Can you work these out from the model? Positions are in its coordinate system, mm. A direction names the side the tool comes from. Coordinates: 2 decimals unless noted, no trailing zeros. Order: outer loops, then holes, each group sorted by start corner. A loop starts at its lowest first (then second) coordinate and runs counter-clockwise, first axis right, second up. Notation, with made-up numbers: (70, -31) -> (121, -31) arc R25 ccw to (121, -11) -> close; hole circle Ø3 at (-24.75, 27.5). An arc over 180 degrees is marked (long way). Write item = value, one per line.
Autodesk Inventor part; units mm, degrees
ref_plane "YZ Plane" through (0, 0, 0) normal (1, 0, 0) x (0, 1, 0)
ref_plane "XZ Plane" through (0, 0, 0) normal (0, 1, 0) x (-1, 0, 0)
ref_plane "XY Plane" through (0, 0, 0) normal (0, 0, 1) x (1, 0, 0)
sketch "Sketch1" plane through (0, 0, 0) normal (0, 0, 1) x (1, 0, 0)
  line L0 (-81.5, 70) -> (81.5, 70)
  line L1 (81.5, 70) -> (81.5, -70)
  line L2 (81.5, -70) -> (-81.5, -70)
  line L3 (-81.5, -70) -> (-81.5, 70)
  line L4 (-81.5, 70) -> (81.5, -70) construction
  line L5 (81.5, 70) -> (-81.5, -70) construction
  line L6 (81.5, 62) -> (89.5, 62)
  line L7 (89.5, 62) -> (89.5, 44)
  line L8 (89.5, 44) -> (81.5, 44)
  line L9 (81.5, 44) -> (81.5, 62)
  line L10 (81.5, -58) -> (89.5, -58)
  line L11 (89.5, -58) -> (89.5, -40)
  line L12 (89.5, -40) -> (81.5, -40)
  line L13 (81.5, -40) -> (81.5, -58)
  line L14 (-81.5, 62) -> (-89.5, 62)
  line L15 (-89.5, 62) -> (-89.5, 44)
  line L16 (-89.5, 44) -> (-81.5, 44)
  line L17 (-81.5, 44) -> (-81.5, 62)
  line L18 (-81.5, -58) -> (-89.5, -58)
  line L19 (-89.5, -58) -> (-89.5, -40)
  line L20 (-89.5, -40) -> (-81.5, -40)
  line L21 (-81.5, -40) -> (-81.5, -58)
  point P0 (0, 0)
  dimension "d0" = 163
  dimension "d1" = 140
  dimension "d2" = 8
  dimension "d3" = 18
  dimension "d4" = 8
  dimension "d5" = 12
extrude "Extrusion1" add sketch "Sketch1" along normal blind 5
sketch "Sketch2" plane through (0, 0, 5) normal (0, 0, 1) x (1, 0, 0)
  line L0 (-80, -67) -> (80, -67)
  line L1 (80, -67) -> (80, 67)
  line L2 (80, 67) -> (-80, 67)
  line L3 (-80, 67) -> (-80, -67)
  line L4 (-80, -67) -> (80, 67) construction
  line L5 (80, -67) -> (-80, 67) construction
  line L6 (81.5, 70) -> (-81.5, 70)
  line L7 (81.5, -40) -> (81.5, 44)
  point P0 (0, 0)
  dimension "d48" = 160
  dimension "d49" = 134
extrude "Extrusion2" add sketch "Sketch2" along normal blind 11
sketch "Sketch3" plane through (0, 0, 0) normal (1, 0, 0) x (0, 1, 0)
  line L0 (49.75, 0) -> (-49.75, 0)
  line L1 (49.75, 0) -> (66.532, 20)
  line L2 (66.532, 20) -> (-66.532, 20)
  line L3 (-66.532, 20) -> (-49.75, 0)
  point P0 (0, 0)
  point P1 (0, 0)
  dimension "d12" = 99.5
  dimension "d13" = 20
  dimension "d14" = 130
  dimension "d15" = 130
extrude "Extrusion3" cut sketch "Sketch3" against normal mid plane 148
chamfer "Chamfer1" distance 2.82 angle 80 1 edges at (74, 0, 16) measured on face at (78, -21.0585, 16)
chamfer "Chamfer2" distance 2.82 angle 80 1 edges at (-74, 0, 16) measured on face at (-78, 21.0585, 16)
fillet "Fillet1" radius 4 4 edges at (-80, 67, 10.5) (-80, -67, 10.5) (80, 67, 10.5) (80, -67, 10.5)
fillet "Fillet3" radius 1 4 edges at (-75.41, -56.4657, 8.0035) (75.41, -56.4657, 8.0035) (75.41, 56.4657, 8.0035) (-75.41, 56.4657, 8.0035)
fillet "Fillet4" radius 3 8 edges at (89.5, 62, 2.5) (89.5, -40, 2.5) (89.5, -58, 2.5) (89.5, 44, 2.5) (-89.5, 62, 2.5) (-89.5, 44, 2.5) (-89.5, -40, 2.5) (-89.5, -58, 2.5)
fillet "Fillet5" radius 2 12 edges at (-81.5, 70, 2.5) (81.5, 70, 2.5) (-81.5, -70, 2.5) (81.5, -70, 2.5) (-81.5, -58, 2.5) (-81.5, 44, 2.5) (81.5, -40, 2.5) (81.5, -58, 2.5) (81.5, 62, 2.5) (-81.5, 62, 2.5) (-81.5, -40, 2.5) (81.5, 44, 2.5)
sketch "Sketch4" plane through (0, 0, 5) normal (0, 0, 1) x (1, 0, 0)
  line L0 (-84, -50.9) -> (84, -50.9)
  line L1 (84, -50.9) -> (84, 50.9)
  line L2 (84, 50.9) -> (-84, 50.9)
  line L3 (-84, 50.9) -> (-84, -50.9)
  line L4 (-84, -50.9) -> (84, 50.9) construction
  line L5 (84, -50.9) -> (-84, 50.9) construction
  line L6 (-89.5, 59) -> (-89.5, 47)
  line L7 (89.5, 47) -> (89.5, 59)
  line L8 (89.5, -55) -> (89.5, -43)
  line L9 (-89.5, -43) -> (-89.5, -55)
  line L10 (76, 67) -> (-76, 67)
  point P0 (0, 0)
  point P1 (-84, 52.5)
  point P2 (84, 53)
  point P3 (84, -49.5)
  point P4 (-84, -49.5)
  point P5 (89.5, 53)
  dimension "d30" = 168
  dimension "d38" = 102
  dimension "d39" = 101.8
  dimension "d50" = 14.5
hole "Hole1" at (-84, 52.5, 5) at (84, 53, 5) at (84, -49.5, 5) at (-84, -49.5, 5) direction (0, 0, -1) diameter 5.2 end through all
sketch "Sketch5" plane through (0, 0, 0) normal (0, 0, -1) x (-1, 0, 0)
  line L0 (-96.4, 58.75) -> (96.4, 58.75)
  line L1 (96.4, 58.75) -> (96.4, -58.75)
  line L2 (96.4, -58.75) -> (-96.4, -58.75)
  line L3 (-96.4, -58.75) -> (-96.4, 58.75)
  line L4 (-96.4, 58.75) -> (96.4, -58.75) construction
  line L5 (96.4, 58.75) -> (-96.4, -58.75) construction
  circle A0 centre (-84, -49.5) radius 2.6
  circle A1 centre (84, 52.5) radius 2.6
  circle A2 centre (-84, 53) radius 2.6
  circle A3 centre (84, -49.5) radius 2.6
  line L6 (-74, -49.75) -> (-74, 49.75)
  line L7 (-74, 49.75) -> (74, 49.75)
  line L8 (74, 49.75) -> (74, -49.75)
  line L9 (74, -49.75) -> (-74, -49.75)
  arc A4 (-81.5, -68) -> (-79.5, -70) centre (-79.5, -68) ccw
  line L10 (79.5, -70) -> (-79.5, -70)
  arc A5 (79.5, -70) -> (81.5, -68) centre (79.5, -68) ccw
  line L11 (81.5, -60) -> (81.5, -68)
  arc A6 (83.5, -58) -> (81.5, -60) centre (83.5, -60) ccw
  line L12 (86.5, -58) -> (83.5, -58)
  arc A7 (86.5, -58) -> (89.5, -55) centre (86.5, -55) ccw
  line L13 (89.5, -43) -> (89.5, -55)
  arc A8 (89.5, -43) -> (86.5, -40) centre (86.5, -43) ccw
  line L14 (83.5, -40) -> (86.5, -40)
  arc A9 (81.5, -38) -> (83.5, -40) centre (83.5, -38) ccw
  line L15 (81.5, 42) -> (81.5, -38)
  arc A10 (83.5, 44) -> (81.5, 42) centre (83.5, 42) ccw
  line L16 (86.5, 44) -> (83.5, 44)
  arc A11 (86.5, 44) -> (89.5, 47) centre (86.5, 47) ccw
  line L17 (89.5, 59) -> (89.5, 47)
  arc A12 (89.5, 59) -> (86.5, 62) centre (86.5, 59) ccw
  line L18 (83.5, 62) -> (86.5, 62)
  arc A13 (81.5, 64) -> (83.5, 62) centre (83.5, 64) ccw
  line L19 (81.5, 68) -> (81.5, 64)
  arc A14 (81.5, 68) -> (79.5, 70) centre (79.5, 68) ccw
  line L20 (-79.5, 70) -> (79.5, 70)
  arc A15 (-79.5, 70) -> (-81.5, 68) centre (-79.5, 68) ccw
  line L21 (-81.5, 64) -> (-81.5, 68)
  arc A16 (-83.5, 62) -> (-81.5, 64) centre (-83.5, 64) ccw
  line L22 (-86.5, 62) -> (-83.5, 62)
  arc A17 (-86.5, 62) -> (-89.5, 59) centre (-86.5, 59) ccw
  line L23 (-89.5, 47) -> (-89.5, 59)
  arc A18 (-89.5, 47) -> (-86.5, 44) centre (-86.5, 47) ccw
  line L24 (-83.5, 44) -> (-86.5, 44)
  arc A19 (-81.5, 42) -> (-83.5, 44) centre (-83.5, 42) ccw
  line L25 (-81.5, -38) -> (-81.5, 42)
  arc A20 (-83.5, -40) -> (-81.5, -38) centre (-83.5, -38) ccw
  line L26 (-86.5, -40) -> (-83.5, -40)
  arc A21 (-86.5, -40) -> (-89.5, -43) centre (-86.5, -43) ccw
  line L27 (-89.5, -55) -> (-89.5, -43)
  arc A22 (-89.5, -55) -> (-86.5, -58) centre (-86.5, -55) ccw
  line L28 (-83.5, -58) -> (-86.5, -58)
  arc A23 (-81.5, -60) -> (-83.5, -58) centre (-83.5, -60) ccw
  line L29 (-81.5, -68) -> (-81.5, -60)
  point P0 (0, 0)
  point P1 (89.458, -58.5)
  point P2 (-89.458, -58.5)
  point P3 (-89.5, 58.75)
  point P4 (89.5, 58.75)
  point P5 (81.9388, -58.75)
  point P6 (-81.9388, -58.75)
  dimension "d40" = 192.8
  dimension "d41" = 117.5
extrude "Extrusion4" add sketch "Sketch5" along normal blind 6 contours L23 A17 L22 A16 L21 A15 L20 A14 L19 A13 L18 A12 L17 L0 | L2 A6 L11 A5 L10 A4 L29 A23
sketch "Sketch6" plane through (0, 0, -6) normal (0, 0, -1) x (-1, 0, 0)
  line L0 (81.9388, -58.75) -> (-81.9388, -58.75)
  line L1 (-35, -58.75) -> (35, -58.75)
  line L2 (35, -58.75) -> (35, -61.75)
  line L3 (35, -61.75) -> (-35, -61.75)
  line L4 (-35, -61.75) -> (-35, -58.75)
  point P0 (0, 0)
  point P1 (89.458, -58.5)
  point P2 (-89.458, -58.5)
  point P3 (0, -58.75)
  point P4 (35, -58.5)
  dimension "d44" = 3
  dimension "d45" = 70
extrude "Extrusion5" cut sketch "Sketch6" against normal up to surface (6 mm away)
properties part number "DisplayBezel"
Item 1: For faces 1 (the flat face through (81.5, 66, 0)), 2 (the flat face through (1.063, -56.557, 8.112)), 3 (the flat face through (1, 67, 10)), which set-ups out of +Z, -Z, +X, -X, +Y, -Y let a thin tool reach every point of the face, with its end or its side?
A:
face_1 = +Z, -Z, +X, +Y
face_2 = +Z
face_3 = +Z, +X, -X, +Y
Item 2: I want a section at C-C, the plane z = -3. Please give me the cut outline in (x, y).
A:
outline = (-89.5, 58.75) -> (89.5, 58.75) -> (89.5, 59) arc R3 ccw to (86.5, 62) -> (83.5, 62) arc R2 cw to (81.5, 64) -> (81.5, 68) arc R2 ccw to (79.5, 70) -> (-79.5, 70) arc R2 ccw to (-81.5, 68) -> (-81.5, 64) arc R2 cw to (-83.5, 62) -> (-86.5, 62) arc R3 ccw to (-89.5, 59) -> close; (-81.94, -58.75) arc R2 cw to (-81.5, -60) -> (-81.5, -68) arc R2 ccw to (-79.5, -70) -> (79.5, -70) arc R2 ccw to (81.5, -68) -> (81.5, -60) arc R2 cw to (81.94, -58.75) -> (35, -58.75) -> (35, -61.75) -> (-35, -61.75) -> (-35, -58.75) -> close
Item 3: If I drill on probe 1 along Y at (x, z) = (84, 1.7); probe 2 along Y at (x, z) = (-84, 2.5); probe 3 along X at (y, z) = (52.5, 1.15), over which ranges is the centre line in solid material (lowest first)?
A:
probe_1 = -58 to -52.1, -46.9 to -40, 44 to 50.4, 55.6 to 62
probe_2 = -58 to -52.1, -46.9 to -40, 44 to 49.9, 55.1 to 62
probe_3 = -89.5 to -86.6, -81.4 to 81.45, 86.55 to 89.5
Item 4: I'm going to push flat-ended pins straight in: P1, Ø1, axis at x = 27, z = 13, coming from the +Y side; P2, Ø10, axis at x = -35.5, y = -44.5, coming from the +Z side; P3, Ø3.5, axis at x = 23, z = 10, coming from the -Y side; P4, Ø5.5, axis at y = 10.5, z = 1.5, coming from the +X side. Where does each tip first touch, or does it pass through?
A:
P1 = 67
P2 = through
P3 = -67
P4 = 81.5
Item 5: I want a section at D-D, the plane x = 20. Please give me the cut outline in (y, z).
A:
outline = (-70, -6) -> (-61.75, -6) -> (-61.75, 0) -> (-49.75, 0) -> (-63.18, 16) -> (-67, 16) -> (-67, 5) -> (-70, 5) -> close; (49.75, 0) -> (58.75, 0) -> (58.75, -6) -> (70, -6) -> (70, 5) -> (67, 5) -> (67, 16) -> (63.18, 16) -> close
Item 6: If we mould it in two halves opening along X, with no side actions, what happens to faces 4 (the flat face through (89.5, -49, 2)), 5 (the cylindrical face through (-75.115, 55.918, 7.757)), 6 (the cylindrical face through (-78.859, -65.797, 10.577))? For each: pulls with the +X half, pulls with the -X half, needs draft (parallel to the pull), parting line crosses it, or undercut.
A:
face_4 = pulls with the +X half
face_5 = undercut
face_6 = pulls with the -X half
Item 7: I want a section at B-B, the plane x = -50.5. Please give me the cut outline in (y, z).
A:
outline = (-70, -6) -> (-58.75, -6) -> (-58.75, 0) -> (-49.75, 0) -> (-63.18, 16) -> (-67, 16) -> (-67, 5) -> (-70, 5) -> close; (49.75, 0) -> (58.75, 0) -> (58.75, -6) -> (70, -6) -> (70, 5) -> (67, 5) -> (67, 16) -> (63.18, 16) -> close
